For this review, take the finished solid that the model builds, in its own axes (mm). A direction names the side the tool comes from. Coordinates: 2 decimals unless noted, no trailing zeros. Write each loop counter-clockwise with the first axis right and the second up, starting at its lowest first coordinate (ties: lowest second). Pieces come first, ordered by that corner, then holes. Notation, with made-up numbers: (62.25, 57) - (67.25, 57) arc R23 ccw to (67.25, 71) - close; hole circle Ø3 at (-8, 4.5). An arc over 180 degrees is marked (long way). Use one line per item in the form item = value. Start each with the question number.
1) We need section B-B (y = -74). Give the boundary of the cut face in (x, z), plus the area to 3 significant figures.
2) Insertion check: P1, Ø4, axis at x = -265.5, z = 19.5, coming from the -Y side; P2, Ø3, axis at x = -211.5, y = -37.5, coming from the -Z side; P3, Ø13, axis at y = -112.5, z = -18.5, coming from the -X side; P4, Ø5.5, axis at x = -3, z = 16.5, coming from the +Y side. Each pin has a flat end and moves straight along its axis. Give the tip position at first contact, or say it passes through.
3) We need section C-C (z = 31). Give the boundary of the cut face in (x, y), plus the area to 3 significant figures.
4) Tool access review of faces 4 (the flat face through (-2, -43.014, 19)), 5 (the flat face through (-132, -32, 45)), 6 (the flat face through (-131, -7, -3)), 7 (the flat face through (-2, -31, 0)), 8 (the flat face through (-133, -36, 48)): name each direction out of +Z, -Z, +X, -X, +Y, -Y from which nothing blocks a thin tool from reaching the whole face with its end or side.
5) We need section D-D (x = -26.5). Give the boundary of the cut face in (y, z), plus the area to 3 significant figures.
6) For L1, parallel to Z at x = -42, y = -14; L2, parallel to Y at x = -229.5, z = 21; L3, parallel to X at y = -7, z = 5, list the stretches that pass through material, from the lowest coordinate up. Write a range as from..to.
7) We need section A-A (y = -136.4). Give the boundary of the cut face in (x, z).
8) Mouldability with a two-part tool opening along X and no side actions: class faces 1 (the flat face through (-266.6, -40, 25)), 2 (the flat face through (-120.3, -120, -44)), 3 (the flat face through (-163, -143.442, -53)) as pulls with the +X half, pulls with the -X half, needs draft (parallel to the pull), parting line crosses it, or undercut.
```python
from build123d import *

# Parameters (mm, degrees)
SKETCH1_W                     = 5
SKETCH1_H                     = 47.5
SKETCH1_W_2                   = 67
SKETCH1_H_2                   = 5
SKETCH1_H_3                   = 34.5
SKETCH1_H_4                   = 8
WALLS_DEPTH                   = 50
ROOF_START                    = 50
SKETCH1_3_W                   = 266.6000032
SKETCH1_3_H                   = 105
SKETCH1_3_W_2                 = 67
SKETCH1_3_H_2                 = 67
ROOF_DEPTH                    = 5
SKETCH1_4_W                   = 256.6000032
SKETCH1_4_H                   = 5
SKETCH1_4_W_2                 = 5
SPACER_DEPTH                  = 42
FIBER_CUTOUT_DEPTH            = 291.861757036
FIBER_CUTOUT_DEPTH_BACK       = 291.861757036
SKETCH2_W                     = 38
SKETCH2_H                     = 10
M3_CLEARANCE_HOLE_D           = 3.4
SKETCH1_6_W                   = 5
SKETCH1_6_H                   = 8
SKETCH1_6_W_2                 = 256.6000032
REAR_WALL_FLOOR_DEPTH         = 3
WINDOW_THROUGH_CUT_DEPTH      = 291.861757036
WINDOW_THROUGH_CUT_DEPTH_BACK = 70
SKETCH6_W                     = 70
SKETCH6_H                     = 1.5
WINDOW_START                  = 50
SKETCH1_8_W                   = 67
SKETCH1_8_H                   = 47.5
SKETCH1_8_H_2                 = 14.5
WINDOW_SLOT_CUT_DEPTH         = 5
SKETCH1_9_W                   = 67
SKETCH1_9_H                   = 5
WINDOW_EDGE_THROUGH_CUT_DEPTH = 3.5
FRONT_LEG_MOUNTING_DEPTH      = 45
FRONT_LEG_MOUNTING_DEPTH_BACK = 45
F_1_4_CLEARANCE_HOLE1_D       = 6.7564
FRONT_HOLE_CUTOUT_REACH       = 292.129


with BuildPart() as part:
    # Sketch1 → Walls (new body)
    with BuildSketch(Plane(origin=(0, 0, 0), x_dir=(-1, 0, 0), z_dir=(0, 0, 1))):
        Polygon((0, 105), (0, 100), (5, 100), (99.8000016, 100), (99.8000016, 105), align=None)
        Polygon((166.8000016, 100), (261.6000032, 100), (266.6000032, 100), (266.6000032, 105), (166.8000016, 105), align=None)
        with Locations((264.1000032, 76.25)):
            Rectangle(SKETCH1_W, SKETCH1_H)
        with Locations((133.3000016, 102.5)):
            Rectangle(SKETCH1_W_2, SKETCH1_H_2)
        with Locations((264.1000032, 35.25)):
            Rectangle(SKETCH1_W, SKETCH1_H_3)
        with Locations((264.1000032, 15.5)):
            Rectangle(SKETCH1_W, SKETCH1_H_2)
        with Locations((264.1000032, 9)):
            Rectangle(SKETCH1_W, SKETCH1_H_4)
        Polygon((5, 5), (0, 5), (0, 0), (266.6000032, 0), (266.6000032, 5), (261.6000032, 5), align=None)
        with Locations((2.5, 9)):
            Rectangle(SKETCH1_W, SKETCH1_H_4)
        with Locations((2.5, 15.5)):
            Rectangle(SKETCH1_W, SKETCH1_H_2)
        with Locations((2.5, 35.25)):
            Rectangle(SKETCH1_W, SKETCH1_H_3)
        with Locations((2.5, 76.25)):
            Rectangle(SKETCH1_W, SKETCH1_H)
    extrude(amount=WALLS_DEPTH)

    # Sketch1<3> → roof (add)
    with BuildSketch(Plane(origin=(0, 0, 0), x_dir=(-1, 0, 0), z_dir=(0, 0, 1)).offset(ROOF_START)):
        with Locations((133.3000016, 52.5)):
            Rectangle(SKETCH1_3_W, SKETCH1_3_H)
        with Locations((133.3000016, 71.5)):
            Rectangle(SKETCH1_3_W_2, SKETCH1_3_H_2)
    extrude(amount=-ROOF_DEPTH)

    # Sketch1<4> → spacer (add)
    with BuildSketch(Plane(origin=(0, 0, 0), x_dir=(-1, 0, 0), z_dir=(0, 0, 1))):
        with Locations((133.3000016, 15.5)):
            Rectangle(SKETCH1_4_W, SKETCH1_4_H)
        with Locations((2.5, 15.5)):
            Rectangle(SKETCH1_4_W_2, SKETCH1_4_H)
        with Locations((264.1000032, 15.5)):
            Rectangle(SKETCH1_4_W_2, SKETCH1_4_H)
    extrude(amount=-SPACER_DEPTH)

    # Sketch2 → fiber cutout (cut, two sides: drawn at the far end of the back side and taken through both)
    with BuildSketch(Plane.ZY.offset(266.6000032).offset(-FIBER_CUTOUT_DEPTH_BACK)):
        with Locations((19, -48.0141)):
            Rectangle(SKETCH2_W, SKETCH2_H)
    extrude(amount=FIBER_CUTOUT_DEPTH + FIBER_CUTOUT_DEPTH_BACK, mode=Mode.SUBTRACT)

    # M3 Clearance Hole (through all)
    with Locations(Plane.XZ.offset(18)):
        with Locations((-224.6, -9), (-42, -9), (-72, -9), (-72, -37), (-42, -37), (-224.6, -37), (-194.6, -37), (-194.6, -9)):
            Hole(M3_CLEARANCE_HOLE_D / 2)

    # Sketch1<6> → rear wall floor (add)
    with BuildSketch(Plane(origin=(0, 0, 0), x_dir=(-1, 0, 0), z_dir=(0, 0, 1))):
        Polygon((5, 5), (0, 5), (0, 0), (266.6000032, 0), (266.6000032, 5), (261.6000032, 5), align=None)
        with Locations((2.5, 9)):
            Rectangle(SKETCH1_6_W, SKETCH1_6_H)
        with Locations((133.3000016, 9)):
            Rectangle(SKETCH1_6_W_2, SKETCH1_6_H)
        with Locations((264.1000032, 9)):
            Rectangle(SKETCH1_6_W, SKETCH1_6_H)
    extrude(amount=-REAR_WALL_FLOOR_DEPTH)

    # Sketch6 → window through cut (cut, two sides: drawn at the far end of the back side and taken through both)
    with BuildSketch(Plane.XZ.offset(105).offset(-WINDOW_THROUGH_CUT_DEPTH_BACK)):
        with Locations((-133.3000016, 47.25)):
            Rectangle(SKETCH6_W, SKETCH6_H)
    extrude(amount=WINDOW_THROUGH_CUT_DEPTH + WINDOW_THROUGH_CUT_DEPTH_BACK, mode=Mode.SUBTRACT)

    # Sketch1<8> → window slot cut (cut)
    with BuildSketch(Plane(origin=(0, 0, 0), x_dir=(-1, 0, 0), z_dir=(0, 0, 1)).offset(WINDOW_START)):
        with Locations((133.3000016, 76.25)):
            Rectangle(SKETCH1_8_W, SKETCH1_8_H)
        with Locations((133.3000016, 45.25)):
            Rectangle(SKETCH1_8_W, SKETCH1_8_H_2)
    extrude(amount=-WINDOW_SLOT_CUT_DEPTH, mode=Mode.SUBTRACT)

    # Sketch1<9> → window edge through cut (cut)
    with BuildSketch(Plane(origin=(0, 0, 0), x_dir=(-1, 0, 0), z_dir=(0, 0, 1)).offset(WINDOW_START)):
        with Locations((133.3000016, 102.5)):
            Rectangle(SKETCH1_9_W, SKETCH1_9_H)
    extrude(amount=-WINDOW_EDGE_THROUGH_CUT_DEPTH, mode=Mode.SUBTRACT)

    # Sketch7 → Front leg mounting (add, two sides: drawn at the far end of the back side and taken through both)
    with BuildSketch(Plane(origin=(-133.3000016, 0, 50), x_dir=(0, 0, -1), z_dir=(1, 0, 0)).offset(-FRONT_LEG_MOUNTING_DEPTH_BACK)):
        Polygon((105.668753763, -120), (105.668753763, -143.441918177), (100.668753763, -143.441918177), (100.668753763, -123.441918177), (50, -105), (50, -100), (75.668753763, -100), align=None)
    extrude(amount=FRONT_LEG_MOUNTING_DEPTH + FRONT_LEG_MOUNTING_DEPTH_BACK)

    # 1/4 Clearance Hole1 (through all)
    with Locations(Plane.XY.offset(-50.668753763)):
        with Locations((-95.2000016, -136.4), (-171.4000016, -136.4)):
            Hole(F_1_4_CLEARANCE_HOLE1_D / 2)

    # Front hole cutout: up to this face of the body (flat: up to its plane)
    front_hole_cutout_end = Plane(part.part.faces().sort_by_distance((-133.3000016, -143.441918177, -53.168753763))[0])
    # Sketch11 → Front hole cutout (cut, up to the picked face)
    with BuildSketch(Plane(origin=(0, -100, 0), x_dir=(1, 0, 0), z_dir=(0, 1, 0)), mode=Mode.PRIVATE) as front_hole_cutout_sk1:
        Polygon((-146.3000016, 55.668753763), (-146.3000016, 29.5285), (-145.6194242, 25.668753763), (-120.980579, 25.668753763), (-120.3000016, 29.5285), (-120.3000016, 55.668753763), align=None)
    front_hole_cutout_tool1 = split(extrude(front_hole_cutout_sk1.sketch, amount=-FRONT_HOLE_CUTOUT_REACH, mode=Mode.PRIVATE), bisect_by=front_hole_cutout_end, keep=Keep.BOTH, mode=Mode.PRIVATE)
    # Sketch11 → Front hole cutout (cut, up to the picked face)
    with BuildSketch(Plane(origin=(0, -100, 0), x_dir=(1, 0, 0), z_dir=(0, 1, 0)), mode=Mode.PRIVATE) as front_hole_cutout_sk2:
        Polygon((-120.980579, 25.668753763), (-145.6194242, 25.668753763), (-145.065712735, 22.5285), (-121.534290465, 22.5285), align=None)
    front_hole_cutout_tool2 = split(extrude(front_hole_cutout_sk2.sketch, amount=-FRONT_HOLE_CUTOUT_REACH, mode=Mode.PRIVATE), bisect_by=front_hole_cutout_end, keep=Keep.BOTH, mode=Mode.PRIVATE)
    add(front_hole_cutout_tool1.solids().sort_by(Axis((-133.300002, -100, -40.715093), (0, -1, 0)))[0], mode=Mode.SUBTRACT)
    add(front_hole_cutout_tool2.solids().sort_by(Axis((-133.300002, -100, -24.110659), (0, -1, 0)))[0], mode=Mode.SUBTRACT)


solid = part.part
```
Determined:
q1.outline = (-266.6, 0) - (-261.6, 0) - (-261.6, 45) - (-166.8, 45) - (-166.8, 46.5) - (-168.3, 46.5) - (-168.3, 48) - (-166.8, 48) - (-166.8, 50) - (-266.6, 50) - close; (-99.8, 45) - (-5, 45) - (-5, 0) - (0, 0) - (0, 50) - (-99.8, 50) - (-99.8, 48) - (-98.3, 48) - (-98.3, 46.5) - (-99.8, 46.5) - close
q1.area = 1,440 mm²
q2.P1 = -105
q2.P2 = 45
q2.P3 = -178.3
q2.P4 = 0
q3.outline = (-266.6, -105) - (0, -105) - (0, -53.01) - (-5, -53.01) - (-5, -100) - (-261.6, -100) - (-261.6, -53.01) - (-266.6, -53.01) - close; (-266.6, -43.01) - (-261.6, -43.01) - (-261.6, -5) - (-5, -5) - (-5, -43.01) - (0, -43.01) - (0, 0) - (-266.6, 0) - close
q3.area = 3,520 mm²
q4.face_4 = -Z, +X, -X
q4.face_5 = none
q4.face_6 = -Z, +X, -X, +Y
q4.face_7 = -Z, +X, -X, -Y
q4.face_8 = -Y
q5.outline = (-105, 0) - (-100, 0) - (-100, 45) - (-5, 45) - (-5, 0) - (-18, 0) - (-18, -42) - (-13, -42) - (-13, -3) - (0, -3) - (0, 50) - (-105, 50) - close
q5.area = 1,220 mm²
q6.L1 = -42..-38.7, -35.3..-10.7, -7.3..0, 45..50
q6.L2 = -105..-100, -5..0
q6.L3 = -266.6..-261.6, -5..0
q7.outline = (-178.3, -55.67) - (-174.78, -55.67) - (-174.78, -50.67) - (-178.3, -50.67) - close; (-168.02, -55.67) - (-146.3, -55.67) - (-146.3, -50.67) - (-168.02, -50.67) - close; (-120.3, -55.67) - (-98.58, -55.67) - (-98.58, -50.67) - (-120.3, -50.67) - close; (-91.82, -55.67) - (-88.3, -55.67) - (-88.3, -50.67) - (-91.82, -50.67) - close
q8.face_1 = pulls with the -X half
q8.face_2 = undercut
q8.face_3 = needs draft
